For this review, take the finished solid that the model builds, in its own axes (mm). A direction names the side the tool comes from. Round coordinates to 2 decimals unless told otherwise and drop trailing zeros. Write each loop counter-clockwise with the first axis right and the second up, starting at its lowest first coordinate (ties: lowest second). Pieces come first, ordered by that corner, then holes.
from build123d import *

# Parameters (mm, degrees)
F1_DEPTH = 5
F4_DEPTH = 45.5
F5_SIZE  = 0.5


with BuildPart() as f1:
    # F0 (on Top) → F1 (new body)
    with BuildSketch(Plane.XY):
        Polygon((-14.8876575074, 87.1), (-20.4571957112, 87.1), (-22.5358384183, 57.2079033579), (22.5358384183, 57.2079033579), (20.4571957112, 87.1), (14.8876575074, 87.1), (14.8876575074, 93.1), (9.8876575074, 93.1), (9.8876575074, 87.1), (-9.8876575074, 87.1), (-9.8876575074, 93.1), (-14.8876575074, 93.1), align=None)
    extrude(amount=F1_DEPTH)

    # F3 (on offset) → F4 (cut)
    with BuildSketch(Plane.YZ.offset(24.8876575074)):
        with BuildLine():
            Line((95.6, 3), (92.0142135624, 3))
            ThreePointArc((92.0142135624, 3), (90.4708684127, 3.9944313411), (89.1209800542, 2.75))
            Line((89.1209800542, 2.75), (88.1, 2.75))
            Line((88.1, 2.75), (88.1, 2.25))
            Line((88.1, 2.25), (89.1209800542, 2.25))
            ThreePointArc((89.1209800542, 2.25), (90.4708684127, 1.0055686589), (92.0142135624, 2))
            Line((92.0142135624, 2), (95.6, 2))
            Line((95.6, 2), (95.6, 3))
        make_face()
    extrude(amount=-F4_DEPTH, mode=Mode.SUBTRACT)

    # F5
    f5_edges = [f1.edges().sort_by_distance(p)[0] for p in [
        (-12.387658, 93.1, 3),
        (-12.387658, 93.1, 2),
        (12.387658, 93.1, 3),
        (12.387658, 93.1, 2),
    ]]
    chamfer(f5_edges, length=F5_SIZE)


solid = f1.part
(1) We need section A-A, the plane x = -13.5. Give the boundary of the cut face in (y, z), and give its area (3 significant figures).
Geometry check:
outline: (57.21, 0) - (93.1, 0) - (93.1, 1.5) - (92.6, 2) - (92.01, 2) arc R1.5 cw to (89.12, 2.25) - (88.1, 2.25) - (88.1, 2.75) - (89.12, 2.75) arc R1.5 cw to (92.01, 3) - (92.6, 3) - (93.1, 3.5) - (93.1, 5) - (57.21, 5) - close
area: 171 mm2
(2) For pin 1 Ø1.5 at (x, z) = (-1.5, 3.5) entering from +Y, flat-tipped, find the tip position at first contact; note if it passes through.
Geometry check:
pin 1: stops at y = 87.1
(3) Mouldability with a two-part tool opening along Z and no side actions: class faces 1 (the face through (0, 71, 0)), 2 (the face through (12.4, 88.6, 2.25)), 3 (the face through (0, 57.208, 2)), 4 (the face through (-12.4, 88.6, 2.25)) as pulls with the +Z half, pulls with the -Z half, needs draft (parallel to the pull), parting line crosses it, or undercut.
Geometry check:
face 1: pulls with the -Z half
face 2: undercut
face 3: needs draft
face 4: undercut
(4) We need section B-B, the plane y = 67. Give the boundary of the cut face in (x, z).
Geometry check:
outline: (-21.85, 0) - (21.85, 0) - (21.85, 5) - (-21.85, 5) - close
(5) For line 1 along X through (y, z) = (90, 0.6); line 2 along X through (y, z) = (87, 0.9); line 3 along Y through (x, z) = (-16, 0.75), list the stretches that pass through material, from the lowest coordinate up.
Geometry check:
line 1: x = -14.89 to -9.89, 9.89 to 14.89
line 2: x = -20.46 to 20.46
line 3: y = 57.21 to 87.1
(6) For faces 5 (the face through (-14.888, 89, 1)), 6 (the face through (9.888, 89, 1)), 7 (the face through (-12.4, 88.6, 2.75)), 8 (the face through (12.423, 90.498, 3.997)), 9 (the face through (14.888, 89, 1)), list the 3-axis set-ups (+Z, -Z, +X, -X, +Y, -Y) from which the entire face can be reached by the end or side of a thin tool; tool diameter is ignored.
Geometry check:
face 5: +Z, -Z, -X, +Y
face 6: +Z, -Z, +Y
face 7: +X, -X, +Y
face 8: +X, -X
face 9: +Z, -Z, +X, +Y
(7) We need section C-C, the plane x = -2.5. Give the boundary of the cut face in (y, z), and give its area (3 significant figures).
Geometry check:
outline: (57.21, 0) - (87.1, 0) - (87.1, 5) - (57.21, 5) - close
area: 149 mm2
